from build123d import *

# Parameters (mm, degrees)
SKETCH1_R           = 82.55
BOSS_EXTRUDE1_DEPTH = 10
SKETCH2_W           = 30
SKETCH2_H           = 10
CUT_EXTRUDE1_DEPTH  = 13
CUT_EXTRUDE2_START  = -10
CUT_EXTRUDE2_DEPTH  = 10
SKETCH5_W           = 23
SKETCH5_H           = 30
CUT_EXTRUDE4_DEPTH  = 10


with BuildPart() as part:
    # Sketch1 → Boss-Extrude1 (new body)
    with BuildSketch(Plane(origin=(0, 0, 0), x_dir=(1, 0, 0), z_dir=(0, 1, 0))):
        with Locations(Location((0, 0, 0), (0, 0, 270))):
            Circle(SKETCH1_R)
    extrude(amount=BOSS_EXTRUDE1_DEPTH)

    # Sketch2 → Cut-Extrude1 (cut)
    with BuildSketch(Plane(origin=(0, 13, 0), x_dir=(1, 0, 0), z_dir=(0, 1, 0))):
        Rectangle(SKETCH2_W, SKETCH2_H)
    extrude(amount=-CUT_EXTRUDE1_DEPTH, mode=Mode.SUBTRACT)

    # Sketch3 → Cut-Extrude2 (cut)
    with BuildSketch(Plane(origin=(0, 10, 0), x_dir=(1, 0, 0), z_dir=(0, 1, 0)).offset(CUT_EXTRUDE2_START)):
        with BuildLine():
            ThreePointArc((82.55, 0), (0, 82.55), (-82.55, 0))
            Line((-82.55, 0), (-15, 0))
            Line((-15, 0), (-15, 5))
            Line((-15, 5), (15, 5))
            Line((15, 5), (15, 0))
            Line((15, 0), (82.55, 0))
        make_face()
    extrude(amount=CUT_EXTRUDE2_DEPTH, mode=Mode.SUBTRACT)

    # Sketch5 → Cut-Extrude4 (cut)
    with BuildSketch(Plane(origin=(0, 10, 0), x_dir=(1, 0, 0), z_dir=(0, 1, 0))):
        with Locations((26.5, 0)):
            Rectangle(SKETCH5_W, SKETCH5_H)
    extrude(amount=-CUT_EXTRUDE4_DEPTH, mode=Mode.SUBTRACT)


solid = part.part
Can you work these out from the model? Positions are in its coordinate system, mm. A direction names the side the tool comes from. Round coordinates to 2 decimals unless told otherwise and drop trailing zeros. Write each loop counter-clockwise with the first axis right and the second up, starting at its lowest first coordinate (ties: lowest second). Pieces come first, ordered by that corner, then holes. Notation, with made-up numbers: (-30.75, -16) - (-9.75, -16) arc R19 cw to (-9.75, 11) - close; hole circle Ø5 at (22, -25.5). An arc over 180 degrees is marked (long way). Write each question's results on one line, items separated by ' | '. Start each with the question number.
1) Suppose I cut it at B-B (y = 6.25). List the corners of the cut face in (x, z) for me, and give its area (3 significant figures).
2) Please list where these lines run through material, in increasing order: line 1 (Z direction, x = -1, y = 3); line 2 (X direction, y = 7, z = 4.5); line 3 (X direction, y = 3.75, z = 68.5).
3) Which directions (+Z, -Z, +X, -X, +Y, -Y) give clear straight access to the entire face, cutting with the end or side of a thin tool? Please do faces 4 (the flat face through (-49, 5, 0)), 5 (the flat face through (15, 5, 10)).
4) Suppose I cut it at D-D (z = 59.5). List the corners of the cut face in (x, y) for me.
5) We'd pull the mould along X, two halves only. Please class faces 1 (the flat face through (1, 10, 41)), 2 (the cylindrical face through (-1.82, 4.93, 82.53)), 3 (the flat face through (-15, 5, 3)): released by +X, released by -X, zero draft, split by the parting line, or undercut.
6) For pin 1 Ø6 at (y, z) = (2, 30.5) entering from -X; pin 2 Ø2 at (y, z) = (9, 50) entering from +X; pin 3 Ø1.5 at (y, z) = (2.5, 2.5) entering from +X, each with a flat end and sliding along its axis, tell me the tip position at first contact or that it passes through.
7) Suppose I cut it at C-C (x = 0). List the corners of the cut face in (y, z) for me.
8) Suppose I cut it at A-A (z = 12.5). List the corners of the cut face in (x, y) for me, and give its area (3 significant figures).
Here are the results:
1) outline: (-82.55, 0) - (-15, 0) - (-15, 5) - (15, 5) - (15, 15) - (38, 15) - (38, 0) - (82.55, 0) arc R82.55 ccw to start | area: 10,200 mm2
2) line 1: z = 5 to 82.54 | line 2: x = -82.43 to -15, 38 to 82.43 | line 3: x = -46.07 to 46.07
3) face 4: -Z, +X, -X, +Y, -Y | face 5: -Z, +Y, -Y
4) outline: (-57.22, 0) - (57.22, 0) - (57.22, 10) - (-57.22, 10) - close
5) face 1: zero draft | face 2: split by the parting line | face 3: undercut
6) pin 1: stops at x = -77.83 | pin 2: stops at x = 66.43 | pin 3: stops at x = 82.53
7) outline: (0, 5) - (10, 5) - (10, 82.55) - (0, 82.55) - close
8) outline: (-81.6, 0) - (15, 0) - (15, 10) - (-81.6, 10) - close; (38, 0) - (81.6, 0) - (81.6, 10) - (38, 10) - close | area: 1,400 mm2
